Answer from the drawing. Dimensions are ordinates in mm from the lowest x, y and z of the part. Coordinates: 2 decimals unless noted, no trailing zeros. Order: outer loops, then holes, each group sorted by start corner. A loop starts at its lowest first (then second) coordinate and runs counter-clockwise, first axis right, second up.
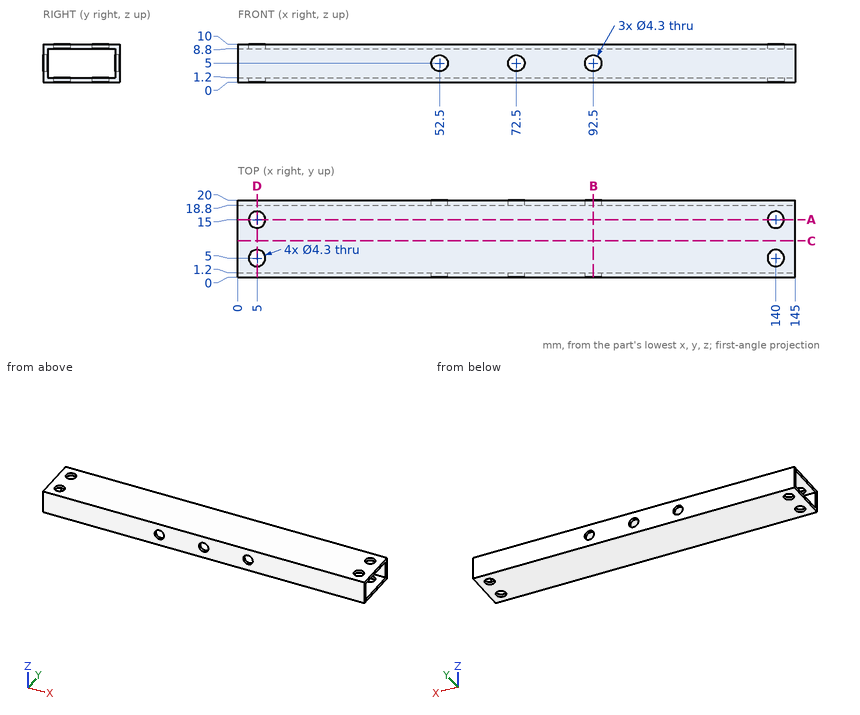
1) Section C-C (y = 9.5) is taken. Give the vertices of the cut face in (x, z).
2) Section A-A (y = 15) is taken. Give the vertices of the cut face in (x, z).
3) Each of these flat-tipped pins is pushed along its axis until it touches: P1, Ø1, axis at y = 17.5, z = 5.5, coming from the -X side; P2, Ø2, axis at y = 4.5, z = 1.5, coming from the -X side. Where does it stop, or does it pass through?
4) Section D-D (x = 5) is taken. Give the vertices of the cut face in (y, z).
5) Section B-B (x = 92.5) is taken. Give the vertices of the cut face in (y, z), then the cut area to 3 significant figures.
6) Consider L1, parallel to X at y = 0.25, z = 5; L2, parallel to Y at x = 140, z = 0.95; L3, parallel to Y at x = 75.5, z = 4.25. Determine where each line is inside the solid, lowest interval first.
Filled sheet:
1. outline: (0, 0) - (145, 0) - (145, 1.2) - (0, 1.2) - close; (0, 8.8) - (145, 8.8) - (145, 10) - (0, 10) - close
2. outline: (0, 0) - (2.85, 0) - (2.85, 1.2) - (0, 1.2) - close; (0, 8.8) - (2.85, 8.8) - (2.85, 10) - (0, 10) - close; (7.15, 0) - (137.85, 0) - (137.85, 1.2) - (7.15, 1.2) - close; (7.15, 8.8) - (137.85, 8.8) - (137.85, 10) - (7.15, 10) - close; (142.15, 0) - (145, 0) - (145, 1.2) - (142.15, 1.2) - close; (142.15, 8.8) - (145, 8.8) - (145, 10) - (142.15, 10) - close
3. P1: passes through
3. P2: stops at x = 0
4. outline: (0, 0) - (2.85, 0) - (2.85, 1.2) - (1.2, 1.2) - (1.2, 8.8) - (2.85, 8.8) - (2.85, 10) - (0, 10) - close; (7.15, 0) - (12.85, 0) - (12.85, 1.2) - (7.15, 1.2) - close; (7.15, 8.8) - (12.85, 8.8) - (12.85, 10) - (7.15, 10) - close; (17.15, 0) - (20, 0) - (20, 10) - (17.15, 10) - (17.15, 8.8) - (18.8, 8.8) - (18.8, 1.2) - (17.15, 1.2) - close
5. outline: (0, 0) - (20, 0) - (20, 2.85) - (18.8, 2.85) - (18.8, 1.2) - (1.2, 1.2) - (1.2, 2.85) - (0, 2.85) - close; (0, 7.15) - (1.2, 7.15) - (1.2, 8.8) - (18.8, 8.8) - (18.8, 7.15) - (20, 7.15) - (20, 10) - (0, 10) - close
5. area: 55.9 mm2
6. L1: x = 0 to 50.35, 54.65 to 70.35, 74.65 to 90.35, 94.65 to 145
6. L2: y = 0 to 2.85, 7.15 to 12.85, 17.15 to 20
6. L3: y = 0 to 1.2, 18.8 to 20
